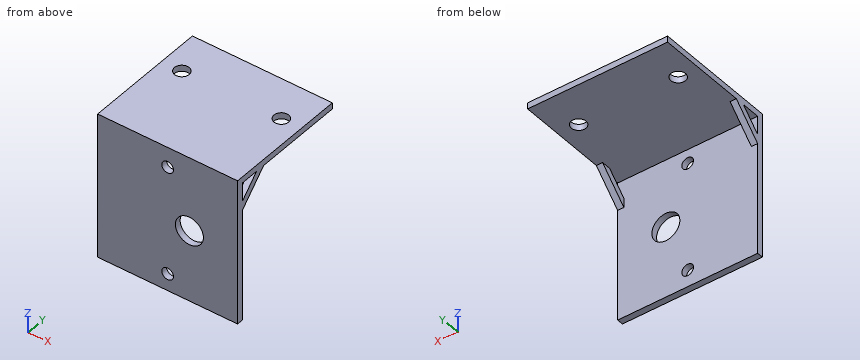
from build123d import *

# Parameters (mm, degrees)
SKETCH7_W           = 45
SKETCH7_H           = 45
SKETCH7_R           = 1.875
SKETCH7_R_2         = 14
SKETCH7_R_3         = 4.5
BOSS_EXTRUDE5_DEPTH = 2
SKETCH7_3_W         = 45
SKETCH7_3_H         = 2
BOSS_EXTRUDE6_DEPTH = 40
BOSS_EXTRUDE7_DEPTH = 2
SKETCH10_R          = 2.375
CUT_EXTRUDE2_DEPTH  = 5


with BuildPart() as part:
    # Sketch7 → Boss-Extrude5 (new body)
    with BuildSketch(Plane(origin=(0, 0, 0), x_dir=(1, 0, 0), z_dir=(0, 1, 0))):
        with Locations((5.756289545, -118.050969126)):
            Rectangle(SKETCH7_W, SKETCH7_H)
        with Locations((5.756289545, -136.050969126)):
            Circle(SKETCH7_R, mode=Mode.SUBTRACT)
        with Locations((5.362034713, -118.985312035)):
            Circle(SKETCH7_R_2, mode=Mode.SUBTRACT)
        with Locations((5.756289545, -101.050969126)):
            Circle(SKETCH7_R, mode=Mode.SUBTRACT)
        with Locations((5.362034713, -118.985312035)):
            Circle(SKETCH7_R_2)
        with Locations((12.756289545, -118.550969126)):
            Circle(SKETCH7_R_3, mode=Mode.SUBTRACT)
    extrude(amount=BOSS_EXTRUDE5_DEPTH)

    # Sketch7_3 → Boss-Extrude6 (add)
    with BuildSketch(Plane(origin=(0, 0, 0), x_dir=(1, 0, 0), z_dir=(0, 1, 0))):
        with Locations((5.756289545, -141.550969126)):
            Rectangle(SKETCH7_3_W, SKETCH7_3_H)
    extrude(amount=BOSS_EXTRUDE6_DEPTH)

    # Sketch8 → Boss-Extrude7 (add)
    with BuildSketch(Plane.ZY.offset(16.743710455)):
        Polygon((140.550969126, 8), (134.550969126, 2), (131.550969126, 2), (140.550969126, 11), align=None)
    boss_extrude7 = extrude(amount=-BOSS_EXTRUDE7_DEPTH)

    # Mirror2: Boss-Extrude7 across plane
    add(boss_extrude7.mirror(Plane.ZY.offset(-5.756289545)))

    # Sketch10 → Cut-Extrude2 (cut)
    with BuildSketch(Plane.XY.offset(142.550969126)):
        with Locations((21.756289545, 27)):
            Circle(SKETCH10_R)
        with Locations((-10.243710455, 27)):
            Circle(SKETCH10_R)
    extrude(amount=-CUT_EXTRUDE2_DEPTH, mode=Mode.SUBTRACT)


solid = part.part
Part model, mm, in its own coordinate system. Give positions to 0.01 mm unless a question says otherwise; leave off trailing zeros. Write each loop counter-clockwise with the first axis right and the second up, starting at its lowest first coordinate (ties: lowest second). Pieces come first, ordered by that corner, then holes.
1) Cut at B-B on x = -4. Write the cut outline in (y, z), then the cut area to 3 significant figures.
Resolved:
outline: (0, 95.55) - (2, 95.55) - (2, 140.55) - (40, 140.55) - (40, 142.55) - (0, 142.55) - close
area: 170 mm2
2) Pin check, flat tips, straight feed: pin 1 (22.5 mm diameter, centred on x = 8.5, z = 111.5, fed in from +Y); pin 2 (4 mm diameter, centred on x = 21.76, y = 27, fed in from -Z) (1 decimal); pin 3 (11.5 mm diameter, centred on x = 4, y = 19.5, fed in from -Z). Stop position of each tip, or through.
Resolved:
pin 1: stops at y = 2
pin 2: passes through
pin 3: stops at z = 140.55
3) Cut at D-D on y = 10. Write the cut outline in (x, z), then the cut area to 3 significant figures.
Resolved:
outline: (-16.74, 139.55) - (-14.74, 139.55) - (-14.74, 140.55) - (26.26, 140.55) - (26.26, 139.55) - (28.26, 139.55) - (28.26, 142.55) - (-16.74, 142.55) - close
area: 94.0 mm2
4) Probe L1, parallel to Z at x = -5.5, y = 16.5; L2, parallel to Y at x = 13, z = 138; L3, parallel to Y at x = -15, z = 135.5. List the from-to ranges inside material, lowest first.
Resolved:
L1: z = 140.55 to 142.55
L2: y = 0 to 2
L3: y = 0 to 2, 2.95 to 5.95
5) Cut at A-A on y = 27. Write the cut outline in (x, z), then the cut area to 3 significant figures.
Resolved:
outline: (-16.74, 140.55) - (-12.62, 140.55) - (-12.62, 142.55) - (-16.74, 142.55) - close; (-7.87, 140.55) - (19.38, 140.55) - (19.38, 142.55) - (-7.87, 142.55) - close; (24.13, 140.55) - (28.26, 140.55) - (28.26, 142.55) - (24.13, 142.55) - close
area: 71.0 mm2
6) Cut at C-C on z = 113. Write the cut outline in (x, y).
Resolved:
outline: (-16.74, 0) - (28.26, 0) - (28.26, 2) - (-16.74, 2) - close
